Can you work these out from the model? Positions are in its coordinate system, mm. A direction names the side the tool comes from. Round coordinates to 2 decimals unless told otherwise and drop trailing zeros. Write each loop counter-clockwise with the first axis right and the second up, starting at its lowest first coordinate (ties: lowest second). Pieces come first, ordered by that corner, then holes.
Q1. If we section it at B-B (x = 8): Please give me the cut outline in (y, z), plus the area to 3 significant figures.
Q2. If we section it at D-D (x = 17): Please give me the cut outline in (y, z), plus the area to 3 significant figures.
Q3. If we section it at A-A (z = 47): Please give me the cut outline in (x, y), plus the area to 3 significant figures.
Q4. Please list where these lines run through material, in increasing order: line 1 along Y through (x, z) = (17, 40.5); line 2 along X through (y, z) = (-12, 21); line 3 along Z through (x, y) = (-10, 6.5).
Q5. We'd pull the mould along Z, two halves only. Please class faces 1 (the cylindrical face through (13.446, 19.241, 31.1)), 2 (the flat face through (-9, -15, 50)), 3 (the cylindrical face through (7.9, -16.2, 28.4)), 4 (the flat face through (-36.037, 1, 25)): +Z half, -Z half, draft (parallel to the pull), parting line (faces both ways), or undercut.
Q6. If we section it at C-C (y = -11): Please give me the cut outline in (x, z).
Q7. For faces 5 (the flat face through (-7, 2, 0)), 6 (the flat face through (-33.037, 1, 26)), which set-ups out of +Z, -Z, +X, -X, +Y, -Y let a thin tool reach every point of the face, with its end or its side?
Q8. I'm going to push a flat-ended pin straight in: pin 1 Ø3 at (x, y) = (5, 13.5) entering from -Z. Where does the tip first touch, or does it pass through?
from build123d import *

# Parameters (mm, degrees)
F0_W     = 57.9878091812
F0_H     = 38.4146366268
F1_DEPTH = 50
F2_T     = -3
F4_DEPTH = 38.4156366268


with BuildPart() as f1:
    # F0 (on Top) → F1 (new body)
    with BuildSketch(Plane.XY):
        with Locations((-7.042683661, 1.5548774973)):
            Rectangle(F0_W, F0_H)
    extrude(amount=F1_DEPTH)

    # F2
    f2_openings = [f1.faces().sort_by_distance(p)[0] for p in [
        (-7.042684, 1.554877, 50),
    ]]
    offset(amount=F2_T, openings=f2_openings)

    # F3 (on face) → F4 (cut, through all)
    with BuildSketch(Plane.XZ.offset(17.6524408162)):
        with BuildLine():
            add(Edge.make_bspline(
                [(-16.4634156972, 37.4085381627), (-11.1890363739, 34.5487939189), (1.3150993888, 26.6227449202), (-21.2683478099, 12.525752902), (-22.3954826963, 30.3245935739), (-27.2033055371, 42.5719243048), (-20.3772871456, 39.5306212856), (-16.4634156972, 37.4085381627)],
                knots=[0, 0, 0, 0, 0.2260787274, 0.4448680265, 0.65498218, 0.8322374972, 1, 1, 1, 1], degree=3))
        make_face()
        with BuildLine():
            ThreePointArc((15.1829272509, 22.5914642215), (13.3867242374, 31.2103747375), (7.1341460571, 37.4085381627))
            ThreePointArc((7.1341460571, 37.4085381627), (7.9688071733, 28.2673085728), (15.1829272509, 22.5914642215))
        make_face()
    extrude(amount=-F4_DEPTH, mode=Mode.SUBTRACT)


solid = f1.part
A:
1. outline: (-17.65, 0) - (20.76, 0) - (20.76, 28.21) - (17.76, 28.21) - (17.76, 3) - (-14.65, 3) - (-14.65, 28.21) - (-17.65, 28.21) - close; (-17.65, 36.91) - (-14.65, 36.91) - (-14.65, 50) - (-17.65, 50) - close; (17.76, 36.91) - (20.76, 36.91) - (20.76, 50) - (17.76, 50) - close
1. area: 345 mm2
2. outline: (-17.65, 0) - (20.76, 0) - (20.76, 50) - (17.76, 50) - (17.76, 3) - (-14.65, 3) - (-14.65, 50) - (-17.65, 50) - close
2. area: 397 mm2
3. outline: (-36.04, -17.65) - (21.95, -17.65) - (21.95, 20.76) - (-36.04, 20.76) - close; hole (-33.04, -14.65) - (18.95, -14.65) - (18.95, 17.76) - (-33.04, 17.76) - close
3. area: 542 mm2
4. line 1: y = -17.65 to -14.65, 17.76 to 20.76
4. line 2: x = -36.04 to -33.04, 18.95 to 21.95
4. line 3: z = 0 to 3
5. face 1: undercut
5. face 2: +Z half
5. face 3: undercut
5. face 4: draft
6. outline: (-36.04, 0) - (21.95, 0) - (21.95, 50) - (18.95, 50) - (18.95, 3) - (-33.04, 3) - (-33.04, 50) - (-36.04, 50) - close
7. face 5: -Z, +X, -X, +Y, -Y
7. face 6: +Z
8. pin 1: stops at z = 0
